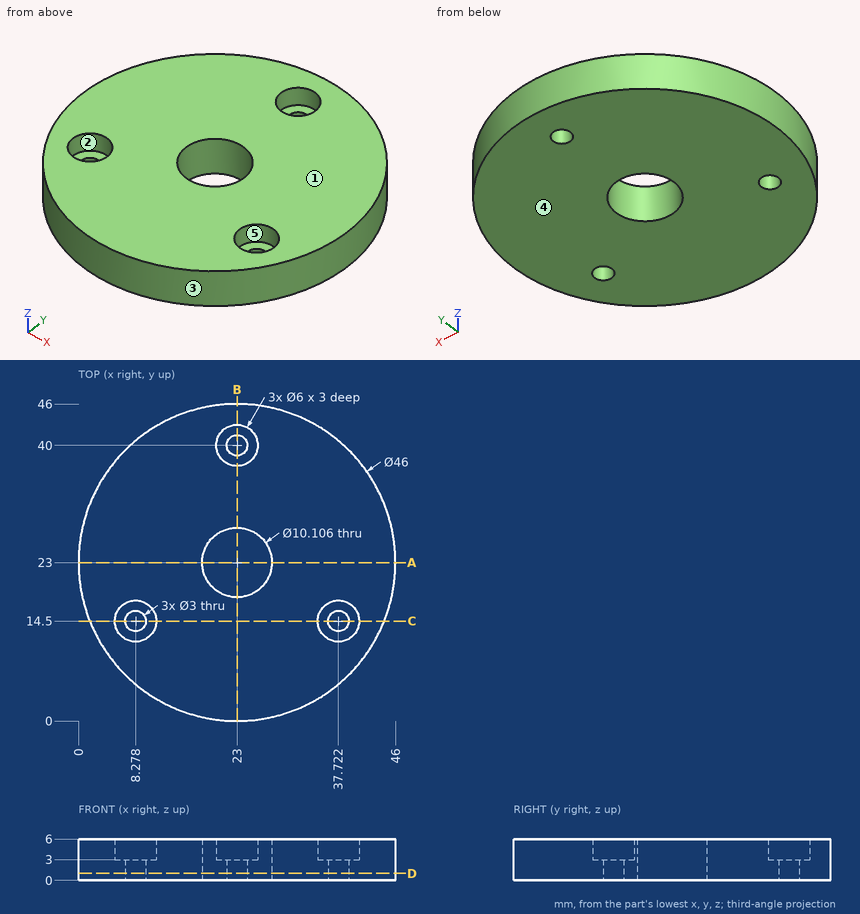
For this review, use the dimensioned drawing (mm, ordinates from the lowest corner) and the shaded views. A direction names the side the tool comes from. Round coordinates to 2 decimals unless told otherwise and drop trailing zeros. Order: outer loops, then holes, each group sorted by start corner. A loop starts at its lowest first (then second) coordinate and runs counter-clockwise, first axis right, second up. Notation, with made-up numbers: (-31.5, 30.25) -> (-26.5, 30.25) arc R27 cw to (-26.5, 65.25) -> close; hole circle Ø11 at (64.5, -1.75). An arc over 180 degrees is marked (long way). Use CSV: the item, a comma, the result in double quotes. Start each with the question number.
(1) Wall thickness on probe 1 along Y at (x, z) = (23, 5.1); probe 2 along X at (y, z) = (14.5, 1.85); probe 3 along X at (y, z) = (14.5, 4.4): over which ranges is each line inside the solid? List them lowest first. Write a range as from..to.
(2) Consider section A-A on y = 23. Write out the cut boundary in (x, z), and give its area (3 significant figures).
(3) Insertion check: pin 1 (1.8 mm diameter, centred on x = 8.28, y = 14.5, fed in from +Z); pin 2 (1.5 mm diameter, centred on x = 16, z = 2.5, fed in from +Y) (1 decimal); pin 3 (1.8 mm diameter, centred on x = 22, y = 39.5, fed in from +Z). Each pin has a flat end and moves straight along its axis. Give the tip position at first contact, or say it passes through.
(4) Consider section D-D on z = 1. Write out the cut boundary in (x, y).
(5) Consider section B-B on x = 23. Write out the cut boundary in (y, z), and give its area (3 significant figures).
(6) Consider section C-C on y = 14.5. Write out the cut boundary in (x, z).
(7) Tool access review of the marked faces 4 and 5: name each direction out of +Z, -Z, +X, -X, +Y, -Y from which nothing blocks a thin tool from reaching the whole face with its end or side.
(8) Mouldability with a two-part tool opening along X and no side actions: class the marked faces 1, 2 and 3 as pulls with the +X half, pulls with the -X half, needs draft (parallel to the pull), parting line crosses it, or undercut.
Responses:
1,probe 1,"0..17.95, 28.05..37, 43..46"
1,probe 2,"1.63..6.78, 9.78..36.22, 39.22..44.37"
1,probe 3,"1.63..5.28, 11.28..34.72, 40.72..44.37"
2,outline,"(0, 0) -> (17.95, 0) -> (17.95, 6) -> (0, 6) -> close; (28.05, 0) -> (46, 0) -> (46, 6) -> (28.05, 6) -> close"
2,area,"215 mm²"
3,pin 1,"through"
3,pin 2,"y = 45.1"
3,pin 3,"z = 3"
4,outline,"circle Ø46 at (23, 23); hole circle Ø3 at (8.28, 14.5); hole circle Ø10.11 at (23, 23); hole circle Ø3 at (23, 40); hole circle Ø3 at (37.72, 14.5)"
5,outline,"(0, 0) -> (17.95, 0) -> (17.95, 6) -> (0, 6) -> close; (28.05, 0) -> (38.5, 0) -> (38.5, 3) -> (37, 3) -> (37, 6) -> (28.05, 6) -> close; (41.5, 0) -> (46, 0) -> (46, 6) -> (43, 6) -> (43, 3) -> (41.5, 3) -> close"
5,area,"188 mm²"
6,outline,"(1.63, 0) -> (6.78, 0) -> (6.78, 3) -> (5.28, 3) -> (5.28, 6) -> (1.63, 6) -> close; (9.78, 0) -> (36.22, 0) -> (36.22, 3) -> (34.72, 3) -> (34.72, 6) -> (11.28, 6) -> (11.28, 3) -> (9.78, 3) -> close; (39.22, 0) -> (44.37, 0) -> (44.37, 6) -> (40.72, 6) -> (40.72, 3) -> (39.22, 3) -> close"
7,face 4,"-Z, +X, -X, +Y, -Y"
7,face 5,"+Z"
8,face 1,"needs draft"
8,face 2,"undercut"
8,face 3,"parting line crosses it"
